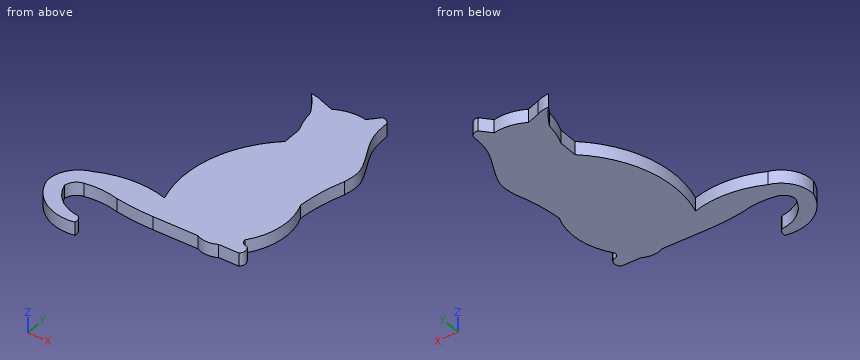
from build123d import *

# Parameters (mm, degrees)
F1_DEPTH = 7.62


with BuildPart() as f1:
    # F0 (on Top) → F1 (new body)
    with BuildSketch(Plane.XY):
        with BuildLine():
            Line((23.0912789702, 76.0052353144), (17.8084038198, 70.2963247895))
            ThreePointArc((17.8084038198, 70.2963247895), (8.6634944394, 70.6002323484), (0, 67.6564946771))
            Line((0, 67.6564946771), (-7.3704631068, 70.2963247895))
            ThreePointArc((-7.3704631068, 70.2963247895), (-10.9539259189, 71.6101956409), (-14.7409262136, 72.085686028))
            ThreePointArc((-14.7409262136, 72.085686028), (-10.213242371, 66.1021431066), (-6.3905753195, 59.6453696489))
            ThreePointArc((-6.3905753195, 59.6453696489), (-5.0838681181, 52.3672612966), (-2.8118535411, 45.3304797411))
            Line((-2.8118535411, 45.3304797411), (-2.8118535411, 41.7517572641))
            Line((-2.8118535411, 41.7517572641), (-2.8118535411, 34.2534817755))
            ThreePointArc((-2.8118535411, 34.2534817755), (-23.1818973657, 2.6551564858), (-22.5800313056, -34.9351428449))
            ThreePointArc((-22.5800313056, -34.9351428449), (-42.6842106724, -32.6463068594), (-62.2868053615, -37.6617908478))
            ThreePointArc((-62.2868053615, -37.6617908478), (-72.2180153419, -44.540137131), (-75.2383731306, -56.2370605767))
            ThreePointArc((-75.2383731306, -56.2370605767), (-64.0161548515, -71.4793290405), (-45.4291552305, -75.0554129481))
            ThreePointArc((-45.4291552305, -75.0554129481), (-45.5811738976, -72.1967918586), (-47.3380211435, -69.9366343501))
            ThreePointArc((-47.3380211435, -69.9366343501), (-59.3231701644, -65.0485814613), (-66.3964748383, -54.208599031))
            ThreePointArc((-66.3964748383, -54.208599031), (-64.3950240146, -49.7065480026), (-60.0098781288, -47.4604927003))
            ThreePointArc((-60.0098781288, -47.4604927003), (-50.2011220543, -46.7688928413), (-40.4885821044, -48.3040064573))
            ThreePointArc((-40.4885821044, -48.3040064573), (-29.4405166496, -49.6518451362), (-18.3196496218, -50.1021072268))
            Line((-18.3196496218, -50.1021072268), (7.583483588, -50.1021072268))
            ThreePointArc((7.583483588, -50.1021072268), (13.5480200406, -51.6228464718), (19.5125564933, -50.1021072268))
            Line((19.5125564933, -50.1021072268), (31.1008002609, -50.1021072268))
            ThreePointArc((31.1008002609, -50.1021072268), (32.6485228526, -46.8642171472), (31.1008002609, -43.6263270676))
            ThreePointArc((31.1008002609, -43.6263270676), (28.4590448896, -42.6406855761), (27.3516643792, -40.0476045907))
            ThreePointArc((27.3516643792, -40.0476045907), (34.956966389, -21.9021038691), (32.4641223997, -2.3858146742))
            ThreePointArc((32.4641223997, -2.3858146742), (34.4601677821, 11.2898780989), (38.2795948535, 24.5722252876))
            add(Edge.make_bspline(
                [(27.5220777839, 73.6194252968), (27.5909354629, 68.6808290163), (27.6540694888, 57.7061514867), (41.4414505958, 37.0315643617), (38.9570749828, 28.2342427003), (38.2795948535, 24.5722252876)],
                knots=[0, 0, 0, 0, 0.3235605926, 0.7188381297, 1, 1, 1, 1], degree=3))
            ThreePointArc((27.5220777839, 73.6194252968), (25.7147995787, 75.5702711821), (23.0912789702, 76.0052353144))
        make_face()
    extrude(amount=F1_DEPTH)


solid = f1.part
Design review of the part built by this model. Coordinates are the model's own, in mm. Round coordinates to 2 decimals unless told otherwise and drop trailing zeros. Write each loop counter-clockwise with the first axis right and the second up, starting at its lowest first coordinate (ties: lowest second). Pieces come first, ordered by that corner, then holes. Notation, with made-up numbers: M 15,-26.5 L 61,-26.5 A26 cw 61,4.5 Z; hole C 69.5,0.5 d11. An arc over 180 degrees is marked long. One line per item, written item: value. Start each with the question number.
1. Clearance check with flat-ended pins moving along their axes: P1, Ø1.5, axis at y = -31.5, z = 3.5, coming from the +X side (3 decimals); P2, Ø2, axis at x = 8, z = 4, coming from the +Y side; P3, Ø4, axis at y = -57, z = 1, coming from the +X side. State where each tip first meets the part, or that it passes through.
2. Take a section at C-C on x = -31. State the section outline as (y, z) points, then the cut area to 3 significant figures.
3. Take a section at A-A on x = -57.5. State the section outline as (y, z) points.
4. To check wall thickness, follow probe 1 along Y at (x, z) = (-14.5, 4.75); probe 2 along Y at (x, z) = (-63, 4.5); probe 3 along X at (y, z) = (13, 6). State the ranges of each line that lie inside material, in increasing order. Write a range as from..to.
5. Take a section at B-B on y = -15.5. State the section outline as (x, z) points.
Computed:
1. P1: stops at x = 32.645
1. P2: stops at y = 70.65
1. P3: stops at x = -64.4
2. outline: M -49.52,0 L -33.07,0 L -33.07,7.62 L -49.52,7.62 Z
2. area: 125 mm²
3. outline: M -74.43,0 L -66.4,0 L -66.4,7.62 L -74.43,7.62 Z; M -47.07,0 L -35.72,0 L -35.72,7.62 L -47.07,7.62 Z
4. probe 1: y = -50.1..21.23, 71.8..72.08
4. probe 2: y = -72.09..-61.16, -48.55..-37.86
4. probe 3: x = -19.24..34.84
5. outline: M -25.67,0 L 35.28,0 L 35.28,7.62 L -25.67,7.62 Z
